```python
from build123d import *

# Parameters (mm, degrees)
SKETCH1_W           = 56
SKETCH1_H           = 36
SKETCH1_R           = 2.4
SKETCH1_W_2         = 42
SKETCH1_H_2         = 22
BOSS_EXTRUDE1_DEPTH = 2.25
CUT_EXTRUDE1_DEPTH  = 2.25


with BuildPart() as part:
    # Sketch1 → Boss-Extrude1 (new body)
    with BuildSketch(Plane(origin=(0, 0, 0), x_dir=(1, 0, 0), z_dir=(0, 1, 0))):
        Rectangle(SKETCH1_W, SKETCH1_H)
        with Locations(Location((24.35, -4.75, 0), (0, 0, 270))):
            Circle(SKETCH1_R, mode=Mode.SUBTRACT)
        with Locations(Location((24.35, 4.75, 0), (0, 0, 270))):
            Circle(SKETCH1_R, mode=Mode.SUBTRACT)
        with Locations(Location((-24.35, -4.75, 0), (0, 0, 270))):
            Circle(SKETCH1_R, mode=Mode.SUBTRACT)
        with Locations(Location((-24.35, 4.75, 0), (0, 0, 270))):
            Circle(SKETCH1_R, mode=Mode.SUBTRACT)
        with Locations(Location((10, 14.5, 0), (0, 0, 270))):
            Circle(SKETCH1_R, mode=Mode.SUBTRACT)
        with Locations(Location((10, -14.5, 0), (0, 0, 270))):
            Circle(SKETCH1_R, mode=Mode.SUBTRACT)
        with Locations(Location((-10, -14.5, 0), (0, 0, 270))):
            Circle(SKETCH1_R, mode=Mode.SUBTRACT)
        with Locations(Location((-10, 14.5, 0), (0, 0, 270))):
            Circle(SKETCH1_R, mode=Mode.SUBTRACT)
        Rectangle(SKETCH1_W_2, SKETCH1_H_2, mode=Mode.SUBTRACT)
    extrude(amount=BOSS_EXTRUDE1_DEPTH)

    # Sketch2 → Cut-Extrude1 (cut)
    with BuildSketch(Plane(origin=(0, 2.25, 0), x_dir=(1, 0, 0), z_dir=(0, 1, 0))):
        Polygon((-28, 11), (-21, 18), (-28, 18), align=None)
        Polygon((-21, -18), (-28, -11), (-28, -18), align=None)
    extrude(amount=-CUT_EXTRUDE1_DEPTH, mode=Mode.SUBTRACT)


solid = part.part
```
Could you check a few things on this model? Use its own coordinates, in mm. A direction names the side the tool comes from. Coordinates: 2 decimals unless noted, no trailing zeros. Write each loop counter-clockwise with the first axis right and the second up, starting at its lowest first coordinate (ties: lowest second). Pieces come first, ordered by that corner, then holes. Notation, with made-up numbers: M -33.75,54 L 10.25,54 A13 ccw 10.25,74 Z; hole C 39.25,29.5 d7. An arc over 180 degrees is marked long. Answer as CSV lines item,"result". Start each with the question number.
1) I want a section at A-A, the plane z = -14.5. Please give me the cut outline in (x, y), and give its area (3 significant figures).
2) I want a section at D-D, the plane z = 4.75. Please give me the cut outline in (x, y).
3) Please list where these lines run through material, in increasing order: line 1 (X direction, y = 1.25, z = -4.75); line 2 (Z direction, x = -3.5, y = 0.75); line 3 (X direction, y = 0.2, z = -0.5). Write a range as from..to.
4) For P1, Ø3, axis at x = 24.35, z = -4.75, coming from the +Y side, with a flat end and sliding along its axis, tell me the tip position at first contact or that it passes through.
5) For faces 1 (the flat face through (-21, 1, 0)), 2 (the flat face through (3, 1, 18)), which set-ups out of +Z, -Z, +X, -X, +Y, -Y let a thin tool reach every point of the face, with its end or its side?
6) I want a section at B-B, the plane x = -24.35. Please give me the cut outline in (y, z), and give its area (3 significant figures).
7) I want a section at C-C, the plane y = 0.95. Give the number of separate pieces and of enclosed holes in the cut face, and give its area (3 significant figures).
Data:
1,outline,"M -24.5,0 L -12.4,0 L -12.4,2.25 L -24.5,2.25 Z; M -7.6,0 L 7.6,0 L 7.6,2.25 L -7.6,2.25 Z; M 12.4,0 L 28,0 L 28,2.25 L 12.4,2.25 Z"
1,area,"96.5 mm^2"
2,outline,"M -28,0 L -26.75,0 L -26.75,2.25 L -28,2.25 Z; M -21.95,0 L -21,0 L -21,2.25 L -21.95,2.25 Z; M 21,0 L 21.95,0 L 21.95,2.25 L 21,2.25 Z; M 26.75,0 L 28,0 L 28,2.25 L 26.75,2.25 Z"
3,line 1,"x = -28..-26.75, -21.95..-21, 21..21.95, 26.75..28"
3,line 2,"z = -18..-11, 11..18"
3,line 3,"x = -28..-21, 21..28"
4,P1,"passes through"
5,face 1,"+Y, -Y"
5,face 2,"+Z, +X, -X, +Y, -Y"
6,outline,"M 0,-14.65 L 2.25,-14.65 L 2.25,-7.15 L 0,-7.15 Z; M 0,-2.35 L 2.25,-2.35 L 2.25,2.35 L 0,2.35 Z; M 0,7.15 L 2.25,7.15 L 2.25,14.65 L 0,14.65 Z"
6,area,"44.3 mm^2"
7,separate pieces,"1"
7,enclosed holes,"9"
7,area,"898 mm^2"
